from build123d import *

# Parameters (mm, degrees)
SKETCH1_R           = 0.425
SKETCH1_R_2         = 0.8
BOSS_EXTRUDE1_DEPTH = 1.6
CUT_EXTRUDE1_DEPTH  = 0.0001
CUT_EXTRUDE2_DEPTH  = 0.0001
PARTFOOTPRINTS_W    = 30.48
PARTFOOTPRINTS_H    = 7.989227112
PARTFOOTPRINTS_W_2  = 3.5
PARTFOOTPRINTS_H_2  = 7.45
CUT_EXTRUDE3_DEPTH  = 0.0001


with BuildPart() as part:
    # Sketch1 → Boss-Extrude1 (new body)
    with BuildSketch(Plane(origin=(0, 0, -0.0125), x_dir=(-1, 0, 0), z_dir=(0, 0, -1))):
        with BuildLine():
            Line((35.3, -50), (35.3, -48))
            ThreePointArc((35.3, -48), (35.592893219, -47.292893219), (36.3, -47))
            Line((36.3, -47), (45.8, -47))
            ThreePointArc((45.8, -47), (46.507106781, -46.707106781), (46.8, -46))
            Line((46.8, -46), (46.8, -41.4))
            ThreePointArc((46.8, -41.4), (47.092893219, -40.692893219), (47.8, -40.4))
            Line((47.8, -40.4), (49.3, -40.4))
            Line((49.3, -40.4), (49.3, 39.2))
            Line((49.3, 39.2), (43.2, 45.3))
            Line((43.2, 45.3), (35.500000002, 45.3))
            Line((35.500000002, 45.3), (35.500000002, 43.8))
            ThreePointArc((35.500000002, 43.8), (35.207106783, 43.092893219), (34.500000002, 42.8))
            Line((34.500000002, 42.8), (4.499999998, 42.8))
            ThreePointArc((4.499999998, 42.8), (3.792893217, 43.092893219), (3.499999998, 43.8))
            Line((3.499999998, 43.8), (3.499999998, 45.3))
            Line((3.499999998, 45.3), (-43.2, 45.3))
            Line((-43.2, 45.3), (-49.3, 39.2))
            Line((-49.3, 39.2), (-49.3, -40.4))
            Line((-49.3, -40.4), (-47.8, -40.4))
            ThreePointArc((-47.8, -40.4), (-47.092893219, -40.692893219), (-46.8, -41.4))
            Line((-46.8, -41.4), (-46.8, -46))
            ThreePointArc((-46.8, -46), (-46.507106781, -46.707106781), (-45.8, -47))
            Line((-45.8, -47), (-36.3, -47))
            ThreePointArc((-36.3, -47), (-35.592893219, -47.292893219), (-35.3, -48))
            Line((-35.3, -48), (-35.3, -50))
            Line((-35.3, -50), (35.3, -50))
        make_face()
        with Locations(Location((-21.27, 40.87, 0), (0, 0, 180))):
            Circle(SKETCH1_R, mode=Mode.SUBTRACT)
        with Locations(Location((-23.81, 40.87, 0), (0, 0, 180))):
            Circle(SKETCH1_R, mode=Mode.SUBTRACT)
        with Locations(Location((-22.54, 39.6, 0), (0, 0, 180))):
            Circle(SKETCH1_R, mode=Mode.SUBTRACT)
        with Locations(Location((-13.87, 40.87, 0), (0, 0, 180))):
            Circle(SKETCH1_R, mode=Mode.SUBTRACT)
        with Locations(Location((-23.81, 38.33, 0), (0, 0, 180))):
            Circle(SKETCH1_R, mode=Mode.SUBTRACT)
        with Locations(Location((-16.41, 40.87, 0), (0, 0, 180))):
            Circle(SKETCH1_R, mode=Mode.SUBTRACT)
        with Locations(Location((-15.14, 39.6, 0), (0, 0, 180))):
            Circle(SKETCH1_R, mode=Mode.SUBTRACT)
        with Locations(Location((-21.27, 38.33, 0), (0, 0, 180))):
            Circle(SKETCH1_R, mode=Mode.SUBTRACT)
        with Locations(Location((-28.67, 40.87, 0), (0, 0, 180))):
            Circle(SKETCH1_R, mode=Mode.SUBTRACT)
        with Locations(Location((-31.21, 40.87, 0), (0, 0, 180))):
            Circle(SKETCH1_R, mode=Mode.SUBTRACT)
        with Locations(Location((-16.41, 38.33, 0), (0, 0, 180))):
            Circle(SKETCH1_R, mode=Mode.SUBTRACT)
        with Locations(Location((-29.94, 39.6, 0), (0, 0, 180))):
            Circle(SKETCH1_R, mode=Mode.SUBTRACT)
        with Locations(Location((-31.21, 38.33, 0), (0, 0, 180))):
            Circle(SKETCH1_R, mode=Mode.SUBTRACT)
        with Locations(Location((-28.67, 38.33, 0), (0, 0, 180))):
            Circle(SKETCH1_R, mode=Mode.SUBTRACT)
        with Locations(Location((33.775, 38.54, 0), (0, 0, 180))):
            Circle(SKETCH1_R_2, mode=Mode.SUBTRACT)
        with Locations((5.225, 38.54)):
            Circle(SKETCH1_R_2, mode=Mode.SUBTRACT)
        with Locations(Location((-13.87, 38.33, 0), (0, 0, 180))):
            Circle(SKETCH1_R, mode=Mode.SUBTRACT)
    extrude(amount=-BOSS_EXTRUDE1_DEPTH)

    # thermalContacts_lower → Cut-Extrude1 (cut)
    with BuildSketch(Plane(origin=(0, 0, -0.0125), x_dir=(-1, 0, 0), z_dir=(0, 0, -1))):
        Polygon((47, 35.5), (47, -41.5), (59.827263463, -41.5), (59.827263463, 47), (41.5, 47), (41.5, 41.5), (41.5, 35.5), align=None)
        Polygon((-47, 35.5), (-47, -41.5), (-56.192158269, -41.5), (-56.192158269, 47), (-41.5, 47), (-41.5, 41.5), (-41.5, 35.5), align=None)
    extrude(amount=-CUT_EXTRUDE1_DEPTH, mode=Mode.SUBTRACT)

    # thermalContacts_upper → Cut-Extrude2 (cut)
    with BuildSketch(Plane.XY.offset(1.5875)):
        Polygon((-47, 35.5), (-47, -41.5), (-56.192158269, -41.5), (-56.192158269, 47), (-41.5, 47), (-41.5, 41.5), (-41.5, 35.5), align=None)
        Polygon((47, 35.5), (47, -41.5), (59.827263463, -41.5), (59.827263463, 47), (41.5, 47), (41.5, 41.5), (41.5, 35.5), align=None)
    extrude(amount=-CUT_EXTRUDE2_DEPTH, mode=Mode.SUBTRACT)

    # partFootprints → Cut-Extrude3 (cut)
    with BuildSketch(Plane.XY.offset(1.5875)):
        with Locations((-19.5, 38.834613556)):
            Rectangle(PARTFOOTPRINTS_W, PARTFOOTPRINTS_H)
        with Locations((15.14, 41.575)):
            Rectangle(PARTFOOTPRINTS_W_2, PARTFOOTPRINTS_H_2)
        with Locations((22.54, 41.575)):
            Rectangle(PARTFOOTPRINTS_W_2, PARTFOOTPRINTS_H_2)
        with Locations((29.94, 41.575)):
            Rectangle(PARTFOOTPRINTS_W_2, PARTFOOTPRINTS_H_2)
    extrude(amount=-CUT_EXTRUDE3_DEPTH, mode=Mode.SUBTRACT)


solid = part.part
Work out the finished part from the listing and answer in its coordinate system (mm). Round coordinates to 2 decimals unless told otherwise and drop trailing zeros. Use one line per item in the form item = value. Start each with the question number.
(1) Consider line 1 (Y direction, x = 16.41, z = 1.2) (3 decimals); line 2 (Y direction, x = 31, z = 0.65); line 3 (Y direction, x = 38.5, z = 0.2). Determine where each line is inside the solid, lowest interval first.
(2) Find section A-A on z = 0.4. Give the number of separate pieces and of enclosed holes in the cut face, and give its area (3 significant figures).
(3) A flat-ended cylindrical pin translates along its axis: P1, Ø0.8, axis at x = 48.5, z = 0.5, coming from the -Y side. Find the tip coordinate at first contact, or state that the pin passes through.
Answer list:
q1.line_1 = -50 to 37.905, 38.755 to 40.445, 41.295 to 45.3
q1.line_2 = -50 to 37.96, 38.7 to 40.5, 41.24 to 45.3
q1.line_3 = -47 to 45.3
q2.separate_pieces = 1
q2.enclosed_holes = 17
q2.area = 9,150 mm^2
q3.P1 = -40.4
